Check sheet for the modelled part. Datum: model origin and axes. Units: mm. A direction names the side the tool comes from. Give positions to 0.01 mm unless a question says otherwise; leave off trailing zeros. Loops run counter-clockwise (first coordinate to the right, second up) from the corner with the lowest first, then second, coordinate; pieces in that order, holes last.
```python
from build123d import *

# Parameters (mm, degrees)
SKETCH1_W                = 15
SKETCH1_H                = 35
REVOLVE1_ANGLE           = 160
SHELL1_T                 = 2
CUT_EXTRUDE4_DEPTH       = 73.816816531
CUT_EXTRUDE4_DEPTH_BACK  = 6
CUT_EXTRUDE5_DEPTH       = 73.816816531
CUT_EXTRUDE5_DEPTH_BACK  = 6
BOSS_EXTRUDE1_START      = -2
SKETCH9_R                = 4.124065783
BOSS_EXTRUDE1_DEPTH      = 2
FILLET4_R                = 3
FILLET5_R                = 3
CUT_EXTRUDE15_DEPTH      = 73.816816664
CUT_EXTRUDE15_DEPTH_BACK = 2
FILLET9_R                = 3


with BuildPart() as part:
    # Sketch1 → Revolve1 (revolve)
    with BuildSketch(Plane(origin=(0, 0, 0), x_dir=(0, 0, -1), z_dir=(1, 0, 0))):
        with Locations((-17.5, 7.5)):
            Rectangle(SKETCH1_W, SKETCH1_H)
    revolve(axis=Axis((0, 25, 25), (0, 0, 1)), revolution_arc=REVOLVE1_ANGLE)

    # Shell1
    shell1_openings = [part.faces().sort_by_distance(p)[0] for p in [
        (0, 7.5, 17.5),
        (5.985352508, 41.444620864, 17.5),
    ]]
    offset(amount=SHELL1_T, openings=shell1_openings, kind=Kind.INTERSECTION)

    # Sketch5 → Cut-Extrude4 (cut, two sides: drawn at the far end of the back side and taken through both)
    with BuildSketch(Plane.XY.offset(27).offset(-CUT_EXTRUDE4_DEPTH_BACK)):
        with BuildLine():
            Line((-139.932865383, 108.358884102), (10.421993206, 53.634190998))
            ThreePointArc((10.421993206, 53.634190998), (30.008933424, 19.708615375), (0, -5.471869593))
            Line((0, -5.471869593), (-160.004298494, -5.471869593))
            Line((-160.004298494, -5.471869593), (-475.151245838, 50.097040112))
            Line((-475.151245838, 50.097040112), (-455.079812728, 163.927793806))
            Line((-455.079812728, 163.927793806), (-139.932865383, 108.358884102))
        make_face()
    extrude(amount=CUT_EXTRUDE4_DEPTH + CUT_EXTRUDE4_DEPTH_BACK, mode=Mode.SUBTRACT)

    # Sketch7 → Cut-Extrude5 (cut, two sides: drawn at the far end of the back side and taken through both)
    with BuildSketch(Plane(origin=(0, 0, 8), x_dir=(-1, 0, 0), z_dir=(0, 0, -1)).offset(-CUT_EXTRUDE5_DEPTH_BACK)):
        Polygon((-42.433629983, 228.653074263), (-12.654745303, 59.768626969), (0, -12), (29.77888468, -180.884447294), (367.547779267, -121.326677934), (295.335264604, 288.210843622), align=None)
    extrude(amount=CUT_EXTRUDE5_DEPTH + CUT_EXTRUDE5_DEPTH_BACK, mode=Mode.SUBTRACT)

    # Sketch9 → Boss-Extrude1 (add)
    with BuildSketch(Plane.XY.offset(27).offset(BOSS_EXTRUDE1_START)):
        with Locations((18.809520277, 48.973668543)):
            Circle(SKETCH9_R)
    extrude(amount=BOSS_EXTRUDE1_DEPTH)

    # Fillet4
    fillet4_edges = [part.edges().sort_by_distance(p)[0] for p in [
        (36.437886861, 18.575017426, 27),
    ]]
    fillet(fillet4_edges, radius=FILLET4_R)

    # Fillet5
    fillet5_edges = [part.edges().sort_by_distance(p)[0] for p in [
        (36.437886861, 18.575017426, 8),
    ]]
    fillet(fillet5_edges, radius=FILLET5_R)

    # Sketch13 → Cut-Extrude15 (cut, two sides: drawn at the far end of the back side and taken through both)
    with BuildSketch(Plane(origin=(0, 0, 8), x_dir=(-1, 0, 0), z_dir=(0, 0, -1)).offset(-CUT_EXTRUDE15_DEPTH_BACK)):
        with BuildLine():
            Line((144.037339106, 25.770763563), (-2.115923769, 0))
            ThreePointArc((-2.115923769, 0), (-30.211686136, 19.672864602), (-10.538821535, 47.768626969))
            Line((-10.538821535, 47.768626969), (135.61444134, 73.539390533))
            Line((135.61444134, 73.539390533), (427.92096709, 125.080917659))
            Line((427.92096709, 125.080917659), (436.343864856, 77.31229069))
            Line((436.343864856, 77.31229069), (144.037339106, 25.770763563))
        make_face()
    extrude(amount=CUT_EXTRUDE15_DEPTH + CUT_EXTRUDE15_DEPTH_BACK, mode=Mode.SUBTRACT)

    # Fillet9
    # the kernel refuses this fillet: 3 mm, written as the material it takes off along each edge
    with BuildSketch(Plane(origin=(6.327372652, 23.884313485, 8), x_dir=(-0.44981568414947964, -0.8931214084843873, 0), z_dir=(-0.8931214084843873, 0.44981568414947964, 0))) as fillet9_piece_1:
        with BuildLine():
            CenterArc((27.081194644, 3), FILLET9_R, 199.471220634, 70.528779366)
            Line((24.252767519, 2), (24.196198976, 1.98))
            ThreePointArc((24.196198976, 1.98), (24.192767519, 1), (24.192767519, 0))
            Line((24.192767519, 0), (24.252767519, -0.06))
            Line((24.252767519, -0.06), (27.081194644, -0.06))
            Line((27.081194644, -0.06), (27.081194644, 0))
        make_face()
    revolve(axis=Axis((6.327372652, 23.884313485, 8), (0, 0, 1)), revolution_arc=213.463718105, mode=Mode.SUBTRACT)


solid = part.part
```
(1) Release check for a two-part mould opening along Z. For faces 1 (the face through (32, 22, 10)), 2 (the face through (36.305, 17.864, 17.409)), 3 (the face through (31, 22, 27)) record: pulls with the +Z half, pulls with the -Z half, needs draft (parallel to the pull), parting line crosses it, or undercut.
(2) Section check A-A on z = 19. Record the boundary of the cut face in (x, y), plus the area to 3 significant figures.
(3) Material ranges on line 1 (Z direction, x = 11, y = -6); line 2 (Y direction, x = 23, z = 21.5); line 3 (Y direction, x = 25, z = 10.5), recorded low to high.
(4) Gauge pin test, flat ends, axial feed: pin 1 Ø0.8 at (x, y) = (12, 59) entering from -Z; pin 2 Ø1 at (x, z) = (30, 12) entering from +Y; pin 3 Ø4 at (y, z) = (2.5, 22.5) entering from -X (3 decimals). Record the tip position at first contact, or that the pin passes through.
(5) Section check B-B on z = 25.75. Record the boundary of the cut face in (x, y), plus the area to 3 significant figures.
(6) Access from +Z, -Z, +X, -X, +Y, -Y to the whole of each face (thin tool, end or side, straight path). Record for faces 4 (the face through (0, -11, 22)), 5 (the face through (34.343, 18.25, 17.395)), 6 (the face through (12.929, 52.593, 25.986)), 7 (the face through (0.838, -7.249, 9.709)).
Computed values:
1. face 1: undercut
1. face 2: needs draft
1. face 3: pulls with the +Z half
2. outline: (0, -12) arc R37 ccw to (12.65, 59.77) - (11.97, 57.89) arc R35 cw to (0, -10) - close
2. area: 201 mm2
3. line 1: z = 8 to 10, 25 to 27
3. line 2: y = -3.98 to -1.38, 51.38 to 53.98
3. line 3: y = -2.22 to 0.51, 49.49 to 52.22
4. pin 1: stops at z = 14
4. pin 2: stops at y = 47.33
4. pin 3: stops at x = 24.995
5. outline: (0, -11.44) arc R36.44 ccw to (12.46, 59.24) - (10.42, 53.63) arc R30.47 cw to (15.4, 51.29) arc R4.12 ccw to (21.87, 46.21) arc R30.47 cw to (0, -5.47) - close
5. area: 583 mm2
6. face 4: +Z, -Z, -X, +Y, -Y
6. face 5: -X
6. face 6: +Z, -X
6. face 7: -Z, -X, +Y
